Build history of the part. All positions in model axes, mm. Round coordinates to 2 decimals unless told otherwise and drop trailing zeros. Order: outer loops, then holes, each group sorted by start corner. A loop starts at its lowest first (then second) coordinate and runs counter-clockwise, first axis right, second up. Notation, with made-up numbers: (-7.75, -18) - (46.25, -18) arc R22 ccw to (46.25, -3) - close; hole circle Ø4 at (-29, 70.25). An arc over 180 degrees is marked (long way). One line per question, with ' | ' between items. Start each with the question number.
Autodesk Inventor part; units mm, degrees
ref_plane "YZ Plane" through (0, 0, 0) normal (1, 0, 0) x (0, 1, 0)
ref_plane "XZ Plane" through (0, 0, 0) normal (0, 1, 0) x (-1, 0, 0)
ref_plane "XY Plane" through (0, 0, 0) normal (0, 0, 1) x (1, 0, 0)
sketch "Sketch8" plane through (0, 0, 0) normal (0, 0, 1) x (1, 0, 0)
  circle A0 centre (0, 0) radius 82
  line L0 (99, -57.1577) -> (0, -114.3154)
  line L1 (0, -114.3154) -> (-99, -57.1577)
  line L2 (-99, -57.1577) -> (-99, 57.1577)
  line L3 (-99, 57.1577) -> (0, 114.3154)
  line L4 (0, 114.3154) -> (99, 57.1577)
  line L5 (99, 57.1577) -> (99, -57.1577)
  dimension "d44" = 164
  dimension "d47" = 198
extrude "Plate3" add sketch "Sketch8" along normal blind 2 contours A0 | L0 L1 L2 L3 L4 L5
equation "\"d48\" = Thickness"
equation "\"BendReliefWidth\" = Thickness"
equation "\"BendReliefDepth\" = 0.5 * Thickness"
equation "\"CornerReliefSize\" = 4 * Thickness"
equation "\"MinimumRemnant\" = 2 * Thickness"
equation "\"TransitionRadius\" = BendRadius"
equation "\"JacobiRadiusSize\" = BendRadius"
equation "\"GapSize\" = Thickness"
equation "\"Octaeder_side\" = d41"
equation "\"Octaeder_flange_lenth\" = d42"
properties part number "DSB 126 hex cup" material "Stainless Steel"
Item 1: Slice it at A-A (z = 0.8). Write the cut outline in (x, y).
Item 2: Slice it at B-B (y = 78). Write the cut outline in (x, z), plus the area to 3 significant figures.
Item 3: Pin check, flat tips, straight feed: pin 1 (1 mm diameter, centred on x = 68, z = 2, fed in from -Y); pin 2 (1 mm diameter, centred on y = 86.5, z = 0.5, fed in from +X). Stop position of each tip, or through.
Item 4: Wall check: line 1 along Y through (x, z) = (14, 1.65); line 2 along Y through (x, z) = (76.5, 0.8); line 3 along X through (y, z) = (66, 0.8). Give the ranges that are in metal, low to high. Write a range as [from, to].
Item 5: Slice it at C-C (x = 39.5). Write the cut outline in (y, z), plus the area to 3 significant figures.
A:
1) outline: (-99, -57.16) - (0, -114.32) - (99, -57.16) - (99, 57.16) - (0, 114.32) - (-99, 57.16) - close
2) outline: (-62.9, 0) - (62.9, 0) - (62.9, 2) - (-62.9, 2) - close | area: 252 mm^2
3) pin 1: y = -75.34 | pin 2: x = 49.04
4) line 1: [-106.23, 106.23] | line 2: [-70.15, 70.15] | line 3: [-83.68, 83.68]
5) outline: (-91.51, 0) - (91.51, 0) - (91.51, 2) - (-91.51, 2) - close | area: 366 mm^2
